Work out the finished part from the listing and answer in its coordinate system (mm). A direction names the side the tool comes from. Round coordinates to 2 decimals unless told otherwise and drop trailing zeros. Loops run counter-clockwise (first coordinate to the right, second up) from the corner with the lowest first, then second, coordinate; pieces in that order, holes last. Notation, with made-up numbers: M -13,-31 L 7,-31 A18 ccw 7,-4 Z; hole C -38.75,59.25 d1. An arc over 180 degrees is marked long. One line per item, written item: value.
```python
from build123d import *

# Parameters (mm, degrees)
SKETCH1_W           = 110
SKETCH1_H           = 110
BOSS_EXTRUDE1_DEPTH = 75
SKETCH2_W           = 100
SKETCH2_H           = 100
CUT_EXTRUDE2_DEPTH  = 70
CUT_EXTRUDE3_START  = -105
CUT_EXTRUDE3_DEPTH  = 105


with BuildPart() as part:
    # Sketch1 → Boss-Extrude1 (new body)
    with BuildSketch(Plane(origin=(0, 0, 0), x_dir=(1, 0, 0), z_dir=(0, 1, 0))):
        Rectangle(SKETCH1_W, SKETCH1_H)
    extrude(amount=BOSS_EXTRUDE1_DEPTH)

    # Sketch2 → Cut-Extrude2 (cut)
    with BuildSketch(Plane(origin=(0, 75, 0), x_dir=(1, 0, 0), z_dir=(0, 1, 0))):
        Rectangle(SKETCH2_W, SKETCH2_H)
    extrude(amount=-CUT_EXTRUDE2_DEPTH, mode=Mode.SUBTRACT)

    # Sketch4 → Cut-Extrude3 (cut)
    with BuildSketch(Plane.XY.offset(55).offset(CUT_EXTRUDE3_START)):
        Polygon((50, 75), (52.294305745, 71.723391823), (-52.294305745, 71.723391823), (-50, 75), align=None)
    extrude(amount=CUT_EXTRUDE3_DEPTH, mode=Mode.SUBTRACT)


solid = part.part
```
1) Find the intervals of material crossed by probe 1 along X at (y, z) = (39.5, -15); probe 2 along Y at (x, z) = (9, -49), in increasing order. Write a range as from..to.
Check values:
probe 1: -55..-50, 50..55
probe 2: 0..5
2) Find section C-C (x = -46). Give the vertices of the cut face in (y, z), then the cut area to 3 significant figures.
Check values:
outline: M 0,-55 L 75,-55 L 75,-50 L 5,-50 L 5,50 L 71.72,50 L 71.72,55 L 0,55 Z
area: 1,230 mm2
3) Find section B-B (z = 13.5). Give the vertices of the cut face in (x, y), then the cut area to 3 significant figures.
Check values:
outline: M -55,0 L 55,0 L 55,75 L 50,75 L 52.29,71.72 L 50,71.72 L 50,5 L -50,5 L -50,71.72 L -52.29,71.72 L -50,75 L -55,75 Z
area: 1,240 mm2
4) For faces 1 (the face through (-1, 37, 55)), 2 (the face through (-1, 39, 50)), determine the directions among +Z, -Z, +X, -X, +Y, -Y from which every point of the face is accessible in a straight line to the end or side of a thin tool.
Check values:
face 1: +Z, +X, -X, +Y, -Y
face 2: +Y
5) The mould has two halves that part along X. Classify faces 3 (the face through (50, 39, 1)), 4 (the face through (55, 37, 1)), 5 (the face through (-1, 37, -55)), 6 (the face through (-55, 37, 1)): +X half, -X half, draft (parallel to the pull), parting line (faces both ways), or undercut.
Check values:
face 3: undercut
face 4: +X half
face 5: draft
face 6: -X half
6) Find section A-A (y = 19). Give the vertices of the cut face in (x, z), then the cut area to 3 significant figures.
Check values:
outline: M -55,-55 L 55,-55 L 55,55 L -55,55 Z; hole M -50,-50 L 50,-50 L 50,50 L -50,50 Z
area: 2,100 mm2
7) This flat-tipped pin is pushed along its axis until it touches: pin 1 (6 mm diameter, centred on x = -3.5, z = 37, fed in from +Y). Where does it stop, or does it pass through?
Check values:
pin 1: y = 5
